Build history of the part. All positions in model axes, mm. Face numbers are marked on the shaded views. A direction names the side the tool comes from. Give positions to 0.01 mm unless a question says otherwise; leave off trailing zeros. Loops run counter-clockwise (first coordinate to the right, second up) from the corner with the lowest first, then second, coordinate; pieces in that order, holes last. Notation, with made-up numbers: (73, -12) - (102, -12) arc R23 cw to (102, -1) - close; hole circle Ø10 at (7.25, 3.5). An arc over 180 degrees is marked (long way). Return JSON: item names as keys, results as strings. Group by question number.
1) Slice it at D-D (y = -53). List the corners of the cut face in (x, z).
2) Drill centre lines: probe 1 along X at (y, z) = (-45.5, 10.75) (3 decimals); probe 2 along Y at (x, z) = (-8.25, 14); probe 3 along Y at (x, z) = (7.25, 17). Where is each one in solid material? Low to high. Write a range as from..to.
3) Slice it at C-C (z = 9.25). List the corners of the cut face in (x, y) (3 decimals), and give its area (3 significant figures).
4) Drop flat-ended pins along their axis: pin 1 (4 mm diameter, centred on x = 2, z = 18, fed in from -Y); pin 2 (1.5 mm diameter, centred on y = -12.5, z = 9.5, fed in from -X) (3 decimals); pin 3 (5.5 mm diameter, centred on y = -13, z = 8, fed in from +X). Give the stop position or say it passes through.
5) Slice it at A-A (y = -25). List the corners of the cut face in (x, z) (3 decimals), and give its area (3 significant figures).
6) Slice it at B-B (x = 0). List the corners of the cut face in (y, z) (3 decimals).
7) 3-axis set-ups, long thin cutter, end or side, ignore diameter. For the marked faces 5, 6 and 7: which of +Z, -Z, +X, -X, +Y, -Y reach the whole face in a straight line?
8) Mould opens along Y. For the marked faces 1, 2, 3 and 4 say: released by +Y, released by -Y, zero draft, split by the parting line, or undercut.
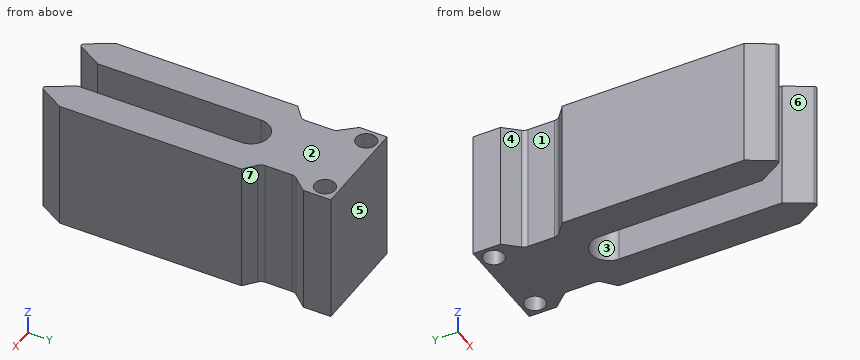
```python
from build123d import *

# Parameters (mm, degrees)
F0_R     = 1.95
F1_DEPTH = 25
F2_R     = 1.5
F3_R     = 0.5


with BuildPart() as f1:
    # F0 (on Top) → F1 (new body)
    with BuildSketch(Plane.XY):
        with BuildLine():
            Line((9.725, 0), (0, 0))
            Line((0, 0), (-9.725, 0))
            Line((-9.725, 0), (-9.725, -5.28))
            Line((-9.725, -5.28), (-6.965, -8.418538))
            Line((-6.965, -8.418538), (-6.965, -14.808538))
            Line((-6.965, -14.808538), (-9.725, -17.13))
            Line((-9.725, -17.13), (-9.725, -52.04))
            Line((-9.725, -52.04), (-6.585, -57.397658))
            Line((-6.585, -57.397658), (-3.445, -52.04))
            Line((-3.445, -52.04), (-3.445, -20.7))
            ThreePointArc((-3.445, -20.7), (0, -17.255), (3.445, -20.7))
            Line((3.445, -20.7), (3.445, -52.04))
            Line((3.445, -52.04), (6.585, -57.397658))
            Line((6.585, -57.397658), (9.725, -52.04))
            Line((9.725, -52.04), (9.725, -17.13))
            Line((9.725, -17.13), (6.965, -14.808538))
            Line((6.965, -14.808538), (6.965, -8.418538))
            Line((6.965, -8.418538), (9.725, -5.28))
            Line((9.725, -5.28), (9.725, 0))
        make_face()
        with Locations((-7.105281, -2.529315)):
            Circle(F0_R, mode=Mode.SUBTRACT)
        with Locations((7.082135, -2.570621)):
            Circle(F0_R, mode=Mode.SUBTRACT)
    extrude(amount=F1_DEPTH)

    # F2
    f2_edges = [f1.edges().sort_by_distance(p)[0] for p in [
        (6.965, -8.418538, 12.5),
        (6.965, -14.808538, 12.5),
        (-6.965, -8.418538, 12.5),
        (-6.965, -14.808538, 12.5),
    ]]
    fillet(f2_edges, radius=F2_R)

    # F3
    f3_edges = [f1.edges().sort_by_distance(p)[0] for p in [
        (-6.585, -57.397658, 12.5),
        (6.585, -57.397658, 12.5),
    ]]
    fillet(f3_edges, radius=F3_R)


solid = f1.part
```
Results:
{
 "1": {"outline": "(-9.16, 0) - (-4.01, 0) - (-4.01, 25) - (-9.16, 25) - close; (4.01, 0) - (9.16, 0) - (9.16, 25) - (4.01, 25) - close"},
 "2": {"probe 1": "-9.725..-3.445, 3.445..9.725", "probe 2": "-54.56..-15.89, -6.96..-4.11, -0.95..0", "probe 3": "-56.26..-14.99, -8.1..-4.51, -0.63..0"},
 "3": {"outline": "(-9.725, -52.04) - (-7.016, -56.662) arc R0.5 ccw to (-6.154, -56.662) - (-3.445, -52.04) - (-3.445, -20.7) arc R3.445 cw to (3.445, -20.7) - (3.445, -52.04) - (6.154, -56.662) arc R0.5 ccw to (7.016, -56.662) - (9.725, -52.04) - (9.725, -17.13) - (7.499, -15.258) arc R1.5 cw to (6.965, -14.11) - (6.965, -8.984) arc R1.5 cw to (7.339, -7.994) - (9.725, -5.28) - (9.725, 0) - (-9.725, 0) - (-9.725, -5.28) - (-7.339, -7.994) arc R1.5 cw to (-6.965, -8.984) - (-6.965, -14.11) arc R1.5 cw to (-7.499, -15.258) - (-9.725, -17.13) - close; hole circle Ø3.9 at (-7.105, -2.529); hole circle Ø3.9 at (7.082, -2.571)", "area": "737 mm2"},
 "4": {"pin 1": "y = -52.99", "pin 2": "x = -6.965", "pin 3": "x = 8.08"},
 "5": {"outline": "(-9.725, 0) - (-3.445, 0) - (-3.445, 25) - (-9.725, 25) - close; (3.445, 0) - (9.725, 0) - (9.725, 25) - (3.445, 25) - close", "area": "314 mm2"},
 "6": {"outline": "(-17.255, 0) - (0, 0) - (0, 25) - (-17.255, 25) - close"},
 "7": {"face 5": "+Z, -Z, +X, -X, +Y", "face 6": "+Z, -Z, -Y", "face 7": "+Z, -Z, +X"},
 "8": {"face 1": "undercut", "face 2": "zero draft", "face 3": "released by -Y", "face 4": "undercut"}
}
